Autodesk Inventor part; units mm, degrees
ref_plane "YZ Plane" through (0, 0, 0) normal (1, 0, 0) x (0, 1, 0)
ref_plane "XZ Plane" through (0, 0, 0) normal (0, 1, 0) x (-1, 0, 0)
ref_plane "XY Plane" through (0, 0, 0) normal (0, 0, 1) x (1, 0, 0)
sketch "Sketch1" plane through (0, 0, 0) normal (0, 0, 1) x (1, 0, 0)
  line L0 (-6.8944, -9.4305) -> (69.3056, -9.4305)
  line L1 (69.3056, -9.4305) -> (69.3056, 41.3695)
  line L2 (69.3056, 41.3695) -> (-6.8944, 41.3695)
  line L3 (-6.8944, 41.3695) -> (-6.8944, -9.4305)
  line L4 (18.5056, 41.3695) -> (43.9056, 41.3695)
  line L5 (43.9056, 41.3695) -> (43.9056, 22.3195)
  line L6 (43.9056, 22.3195) -> (18.5056, 22.3195)
  line L7 (18.5056, 22.3195) -> (18.5056, 41.3695)
  arc A0 (18.5056, 22.3195) -> (43.9056, 22.3195) centre (31.2056, 22.3195) ccw
  point P0 (0, 0)
  point P1 (14.7078, 41.3695)
  point P2 (47.7034, 41.3695)
  point P3 (31.2056, 41.3695)
  dimension "d0" = 76.2
  dimension "d1" = 50.8
  dimension "d6" = 25.4
  dimension "d7" = 19.05
extrude "Extrusion2" add sketch "Sketch1" along normal blind 4.7625 contours L3 L2 L7 A0 L5 L1 L0
sketch "Sketch2" plane through (69.3056, -9.4305, 0) normal (1, 0, 0) x (0, 0, -1)
  line L0 (-4.7625, 50.8) -> (-4.7625, 0)
  line L1 (0, 0) -> (-4.7625, 0)
  line L2 (0, 0) -> (0, 50.8)
  line L3 (0, 50.8) -> (-4.7625, 50.8)
  circle A0 centre (-2.3813, -6.35) radius 6.35
  line L4 (3.7948, -4.8737) -> (0, 11.0013)
  line L5 (-8.5573, -4.8737) -> (-4.7625, 11.0013)
  point P0 (0, 9.4305)
  point P1 (-2.3813, 0)
  dimension "d10" = 12.7
  dimension "d11" = 15.875
extrude "Extrusion3" add sketch "Sketch2" against normal up to surface (76.2 mm away) contours L0 L1 A0 L5 | A0 | L4 A0 L1 L2
sketch "Sketch3" plane through (0, 0, 4.7625) normal (0, 0, 1) x (1, 0, 0)
  arc A0 (18.5056, 22.3195) -> (43.9056, 22.3195) centre (31.2056, 22.3195) ccw
  line L0 (56.6056, -9.4305) -> (56.6056, -22.1305)
  line L1 (5.8056, -22.1305) -> (5.8056, -9.4305)
  line L2 (69.3056, -9.4305) -> (69.3056, -22.1305)
  line L3 (-6.8944, -22.1305) -> (-6.8944, -9.4305)
  line L4 (5.8056, -22.1305) -> (-6.8944, -22.1305)
  line L5 (-6.8944, -9.4305) -> (5.8056, -9.4305)
  line L6 (56.6056, -9.4305) -> (69.3056, -9.4305)
  line L7 (69.3056, -22.1305) -> (56.6056, -22.1305)
  line L8 (12.1556, -9.4305) -> (50.2556, -9.4305)
  line L9 (50.2556, -9.4305) -> (50.2556, -22.1305)
  line L10 (50.2556, -22.1305) -> (12.1556, -22.1305)
  line L11 (12.1556, -22.1305) -> (12.1556, -9.4305)
  point P0 (0, 0)
  point P1 (31.2056, 9.6195)
  point P2 (31.2056, -9.4305)
  dimension "d14" = 50.8
  dimension "d18" = 76.2
  dimension "d19" = 6.35
  dimension "d20" = 6.35
  dimension "d21" = 12.7
  dimension "d22" = 19.05
extrude "Extrusion4" cut sketch "Sketch3" along normal through all both and the other way through all
properties part number "kinect bracket"
Geometry check sheet. Reference: the model listing, model coordinates, mm. A direction names the side the tool comes from. Round coordinates to 2 decimals unless told otherwise and drop trailing zeros. Order: outer loops, then holes, each group sorted by start corner. A loop starts at its lowest first (then second) coordinate and runs counter-clockwise, first axis right, second up. Notation, with made-up numbers: (-3, 39) -> (53, 39) arc R35 ccw to (53, 77) -> close; hole circle Ø2 at (82, -37.75). An arc over 180 degrees is marked (long way). Return JSON: item names as keys, results as strings. Group by question number.
Q1. Tool access check on faces 1 (the flat face through (22, 13, 0)), 2 (the flat face through (50.256, -16, 2)), 3 (the flat face through (56.606, -16, 2)), 4 (the flat face through (18.506, 32, 2)), 5 (the flat face through (-1, -9.43, 2)). Record the directions out of +Z, -Z, +X, -X, +Y, -Y that give a thin tool (end or side, any length) a straight path to the whole face; none if there is none.
Q2. Section check B-B, the plane x = 60. Record the boundary of the cut face in (y, z).
Q3. Release check for a two-part mould opening along X. For faces 6 (the flat face through (5.806, -16, 2)), 7 (the flat face through (43.906, 32, 2)), 8 (the flat face through (22, 13, 4.762)) record: released by +X, released by -X, zero draft, split by the parting line, or undercut.
Q4. Material ranges on probe 1 along X at (y, z) = (-18, 4.75); probe 2 along Z at (x, y) = (38, 10); probe 3 along Y at (x, z) = (17, 2.5), recorded low to high. Write a range as from..to.
Q5. Section check C-C, the plane z = 5.75. Record the boundary of the cut face in (x, y), plus the area to 3 significant figures.
Q6. Gauge pin test, flat ends, axial feed: pin 1 (20 mm diameter, centred on x = 48.5, y = 14.5, fed in from -Z); pin 2 (3 mm diameter, centred on x = 0, z = 4, fed in from -Y); pin 3 (5 mm diameter, centred on x = 49.5, y = -1.5, fed in from +Z). Record the tip position at first contact, or that the pin passes through.
Q7. Section check A-A, the plane y = 33. Record the boundary of the cut face in (x, z), plus the area to 3 significant figures.
Q8. Section check D-D, the plane y = 15. Record the boundary of the cut face in (x, z), plus the area to 3 significant figures.
Numbers:
{
 "1": {"face 1": "-Z, +X, -X, +Y", "face 2": "+Z, -Z, -Y", "face 3": "+Z, -Z, +X, -Y", "face 4": "+Z, -Z, +Y", "face 5": "+Z, -Z, -X, -Y"},
 "2": {"outline": "(-9.43, -2.63) -> (1.57, 0) -> (41.37, 0) -> (41.37, 4.76) -> (1.57, 4.76) -> (-9.43, 7.39) -> close"},
 "3": {"face 6": "released by -X", "face 7": "undercut", "face 8": "zero draft"},
 "4": {"probe 1": "5.81..12.16, 50.26..56.61", "probe 2": "0..4.76", "probe 3": "-9.43..41.37"},
 "5": {"outline": "(-6.89, -9.43) -> (5.81, -9.43) -> (5.81, -21.16) -> (12.16, -21.16) -> (12.16, -9.43) -> (50.26, -9.43) -> (50.26, -21.16) -> (56.61, -21.16) -> (56.61, -9.43) -> (69.31, -9.43) -> (69.31, -2.56) -> (-6.89, -2.56) -> close", "area": "673 mm^2"},
 "6": {"pin 1": "z = 0", "pin 2": "y = -9.43", "pin 3": "z = 6.09"},
 "7": {"outline": "(-6.89, 0) -> (18.51, 0) -> (18.51, 4.76) -> (-6.89, 4.76) -> close; (43.91, 0) -> (69.31, 0) -> (69.31, 4.76) -> (43.91, 4.76) -> close", "area": "242 mm^2"},
 "8": {"outline": "(-6.89, 0) -> (20.83, 0) -> (20.83, 4.76) -> (-6.89, 4.76) -> close; (41.58, 0) -> (69.31, 0) -> (69.31, 4.76) -> (41.58, 4.76) -> close", "area": "264 mm^2"}
}
